```python
from build123d import *

# Parameters (mm, degrees)
SZKIC1_W                    = 224.5
SZKIC1_H                    = 449.9
DODANIE_WYCI_GNI_CIE1_DEPTH = 12.33
SZKIC2_W                    = 219.5
SZKIC2_H                    = 444.9
WYTNIJ_WYCI_GNI_CIE1_DEPTH  = 10
SZKIC4_W                    = 2.5
SZKIC4_H                    = 444.9
WYTNIJ_WYCI_GNI_CIE3_DEPTH  = 5


with BuildPart() as part:
    # Szkic1 → Dodanie-wyciągnięcie1 (new body)
    with BuildSketch(Plane.XY):
        with Locations((112.25, 224.95)):
            Rectangle(SZKIC1_W, SZKIC1_H)
    extrude(amount=DODANIE_WYCI_GNI_CIE1_DEPTH)

    # Szkic2 → Wytnij-wyciągnięcie1 (cut)
    with BuildSketch(Plane(origin=(0, 0, 0), x_dir=(-1, 0, 0), z_dir=(0, 0, -1))):
        with Locations((-112.25, 224.95)):
            Rectangle(SZKIC2_W, SZKIC2_H)
    extrude(amount=-WYTNIJ_WYCI_GNI_CIE1_DEPTH, mode=Mode.SUBTRACT)

    # Szkic4 → Wytnij-wyciągnięcie3 (cut)
    with BuildSketch(Plane(origin=(0, 0, 0), x_dir=(-1, 0, 0), z_dir=(0, 0, -1))):
        with Locations((-223.25, 224.95)):
            Rectangle(SZKIC4_W, SZKIC4_H)
    extrude(amount=-WYTNIJ_WYCI_GNI_CIE3_DEPTH, mode=Mode.SUBTRACT)


solid = part.part
```
Input: part model. Units: mm. Frame: model coordinates. A direction names the side the tool comes from. Coordinates: 2 decimals unless noted, no trailing zeros. Write each loop counter-clockwise with the first axis right and the second up, starting at its lowest first coordinate (ties: lowest second). Pieces come first, ordered by that corner, then holes. Notation, with made-up numbers: (13.5, 51) -> (37.5, 51) arc R18 cw to (37.5, 84) -> close; hole circle Ø5 at (-24.5, 77). An arc over 180 degrees is marked (long way). Write each question's results on one line, items separated by ' | '.
Item 1: Section query B-B on y = 48. Return loops of the section in (x, z).
Conclusion:
outline: (0, 0) -> (2.5, 0) -> (2.5, 10) -> (222, 10) -> (222, 5) -> (224.5, 5) -> (224.5, 12.33) -> (0, 12.33) -> close
Item 2: Material intervals for probe 1 along Y at (x, z) = (145, 5.75); probe 2 along X at (y, z) = (134, 8.25); probe 3 along Z at (x, y) = (11, 202), sorted ascending.
Conclusion:
probe 1: y = 0 to 2.5, 447.4 to 449.9 | probe 2: x = 0 to 2.5, 222 to 224.5 | probe 3: z = 10 to 12.33
Item 3: Mould query, pull axis Y, two halves, no side actions, for faces 3 (the flat face through (0, 222, 6)), 4 (the flat face through (2.5, 222, 5)), 5 (the flat face through (111, 0, 6)), 6 (the flat face through (111, 449.9, 6)). Classes: +Y half, -Y half, draft (parallel to the pull), parting line (faces both ways), or undercut.
Conclusion:
face 3: draft | face 4: undercut | face 5: -Y half | face 6: +Y half
Item 4: Section query A-A on x = 157. Return loops of the section in (y, z), plus the area to 3 significant figures.
Conclusion:
outline: (0, 0) -> (2.5, 0) -> (2.5, 10) -> (447.4, 10) -> (447.4, 0) -> (449.9, 0) -> (449.9, 12.33) -> (0, 12.33) -> close | area: 1,100 mm^2
Item 5: Set-up query: faces 1 (the flat face through (224.5, 222, 9)), 2 (the flat face through (115, 2.5, 5)). Return all of +Z, -Z, +X, -X, +Y, -Y with unobstructed straight access to the full face (end or side cutting, diameter ignored); none if empty.
Conclusion:
face 1: +Z, -Z, +X, +Y, -Y | face 2: -Z
Item 6: Pin query (flat end, axial travel): pin 1 Ø2 at (x, y) = (223.5, 122) entering from -Z; pin 2 Ø6 at (x, y) = (148.5, 100) entering from -Z. Return the tip coordinate at first contact, or that it passes through.
Conclusion:
pin 1: stops at z = 5 | pin 2: stops at z = 10
